Source: CAD feature listing. Evaluate the final solid. Frame: model axes, mm. A direction names the side the tool comes from. Give positions to 0.01 mm unless a question says otherwise; leave off trailing zeros. Order: outer loops, then holes, each group sorted by start corner. A loop starts at its lowest first (then second) coordinate and runs counter-clockwise, first axis right, second up. Notation, with made-up numbers: (19, 8.5) -> (58, 8.5) arc R23 ccw to (58, 33.5) -> close; hole circle Ø7 at (14.5, 10.25). An arc over 180 degrees is marked (long way). Answer in a Markdown table with one row per item.
```python
from build123d import *

# Parameters (mm, degrees)
F0_R     = 8.575
F1_DEPTH = 26.5
F3_DEPTH = 26.5


with BuildPart() as f1:
    # F0 (on Top) → F1 (new body)
    with BuildSketch(Plane.XY):
        Circle(F0_R)
    extrude(amount=F1_DEPTH)

    # F2 (on face) → F3 (cut)
    with BuildSketch(Plane.XY.offset(26.5)):
        Polygon((-0.8024391856, 2.4696538712), (-5.5, 3.995983904), (-2.5967477525, 0), align=None)
        Polygon((2.1008130619, 6.4656377752), (-0.8024391856, 2.4696538712), (2.1008130619, 1.5263300328), align=None)
        Polygon((-0.8024391856, 2.4696538712), (-2.5967477525, 0), (-0.8024391856, -2.4696538712), (2.1008130619, -1.5263300328), (2.1008130619, 1.5263300328), align=None)
        Polygon((-0.8024391856, -2.4696538712), (-2.5967477525, 0), (-5.5, -3.995983904), align=None)
        Polygon((2.1008130619, -1.5263300328), (-0.8024391856, -2.4696538712), (2.1008130619, -6.4656377752), align=None)
        Polygon((6.7983738762, 0), (2.1008130619, 1.5263300328), (2.1008130619, -1.5263300328), align=None)
    extrude(amount=-F3_DEPTH, mode=Mode.SUBTRACT)


solid = f1.part
```
(1) Section query D-D (y = 0.5). Return the cut outline in (x, z), plus the area to 3 significant figures.
A:
| item | result |
|---|---|
| outline | (-8.56, 0) -> (-2.96, 0) -> (-2.96, 26.5) -> (-8.56, 26.5) -> close; (5.26, 0) -> (8.56, 0) -> (8.56, 26.5) -> (5.26, 26.5) -> close |
| area | 236 mm^2 |
(2) First-contact query: pin 1 Ø2 at (x, y) = (2, 5) entering from -Z; pin 2 Ø4 at (x, z) = (-4.5, 16) entering from +Y; pin 3 Ø4 at (y, z) = (5.5, 3.5) entering from -X; pin 4 Ø2 at (y, z) = (-1.5, 7) entering from +X. Flat tips, straight axial feed; report the tip coordinate or a pass-through.
A:
| item | result |
|---|---|
| pin 1 | stops at z = 0 |
| pin 2 | stops at y = 8.2 |
| pin 3 | stops at x = -7.83 |
| pin 4 | stops at x = 8.56 |
(3) Section query C-C (x = -3.5). Return the cut outline in (y, z).
A:
| item | result |
|---|---|
| outline | (-7.83, 0) -> (-3.35, 0) -> (-3.35, 26.5) -> (-7.83, 26.5) -> close; (-1.24, 0) -> (1.24, 0) -> (1.24, 26.5) -> (-1.24, 26.5) -> close; (3.35, 0) -> (7.83, 0) -> (7.83, 26.5) -> (3.35, 26.5) -> close |
(4) Pull-direction query (Y, two-part tool) for faces 3 (the flat face through (-3.184, -3.244, 13.436)), 4 (the cylindrical face through (8.179, 2.576, 13.064)), 5 (the flat face through (0, -4, 0)); classes: +Y half, -Y half, draft (parallel to the pull), parting line (faces both ways), or undercut.
A:
| item | result |
|---|---|
| face 3 | undercut |
| face 4 | parting line |
| face 5 | draft |
(5) Section query A-A (z = 2). Return the cut outline in (x, y) (3 decimals).
A:
| item | result |
|---|---|
| outline | circle Ø17.15 at (0, 0); hole (-5.5, -3.996) -> (-0.802, -2.47) -> (2.101, -6.466) -> (2.101, -1.526) -> (6.798, 0) -> (2.101, 1.526) -> (2.101, 6.466) -> (-0.802, 2.47) -> (-5.5, 3.996) -> (-2.597, 0) -> close |
(6) Section query B-B (y = -3.5). Return the cut outline in (x, z).
A:
| item | result |
|---|---|
| outline | (-7.83, 0) -> (-5.14, 0) -> (-5.14, 26.5) -> (-7.83, 26.5) -> close; (-3.97, 0) -> (-0.05, 0) -> (-0.05, 26.5) -> (-3.97, 26.5) -> close; (2.1, 0) -> (7.83, 0) -> (7.83, 26.5) -> (2.1, 26.5) -> close |
(7) Ray query, probe 1 along Y at (x, z) = (-3, 8.5); probe 2 along Y at (x, z) = (-5.25, 8.25); probe 3 along Y at (x, z) = (-0.5, 9.75). Return the intervals inside material, ascending.
A:
| item | result |
|---|---|
| probe 1 | y = -8.03 to -3.18, -0.56 to 0.56, 3.18 to 8.03 |
| probe 2 | y = -6.78 to -3.91, -3.65 to 3.65, 3.91 to 6.78 |
| probe 3 | y = -8.56 to -2.89, 2.89 to 8.56 |
(8) Access query for faces 1 (the flat face through (0, -4, 26.5)), 2 (the flat face through (4.417, -0.774, 13.436)). Directions: +Z, -Z, +X, -X, +Y, -Y. A direction counts if a zero-diameter tool reaches every point of the face in a straight line with its end or side. Return the directions, or none.
A:
| item | result |
|---|---|
| face 1 | +Z, +X, -X, +Y, -Y |
| face 2 | +Z, -Z |
